```python
from build123d import *

# Parameters (mm, degrees)
SKETCH_1_W          = 100
SKETCH_1_H          = 53
SKETCH_1_W_2        = 30
SKETCH_1_H_2        = 43
SKETCH_1_W_3        = 50
SKETCH_1_H_3        = 25
SKETCH_1_H_4        = 10
EXTRUDE_1_DEPTH     = 7
FILLET_1_R          = 1
CUT_EXTRUDE_2_REACH = 115.393
SKETCH_2_R          = 1.5
SKETCH_3_R          = 1
CUT_EXTRUDE_3_DEPTH = 5


with BuildPart() as part:
    # 草图1 → 凸台-拉伸1 (new body)
    with BuildSketch(Plane.XY):
        with Locations((50, 26.5)):
            Rectangle(SKETCH_1_W, SKETCH_1_H)
        with Locations((20, 26.5)):
            Rectangle(SKETCH_1_W_2, SKETCH_1_H_2, mode=Mode.SUBTRACT)
        with Locations((70, 35.5)):
            Rectangle(SKETCH_1_W_3, SKETCH_1_H_3, mode=Mode.SUBTRACT)
        with Locations((70, 13)):
            Rectangle(SKETCH_1_W_3, SKETCH_1_H_4, mode=Mode.SUBTRACT)
    extrude(amount=EXTRUDE_1_DEPTH)

    # 圆角1
    fillet_1_edges = [part.edges().sort_by_distance(p)[0] for p in [
        (35, 48, 3.5),
        (5, 48, 3.5),
        (5, 5, 3.5),
        (35, 5, 3.5),
        (95, 48, 3.5),
        (45, 48, 3.5),
        (45, 23, 3.5),
        (95, 23, 3.5),
    ]]
    fillet(fillet_1_edges, radius=FILLET_1_R)

    # 草图2 → 切除-拉伸2 (cut, up to next)
    with BuildSketch(Plane.XZ, mode=Mode.PRIVATE) as cut_extrude_2_sk1:
        with Locations(Location((15, 3.5, 0), (0, 0, 270))):
            Circle(SKETCH_2_R)
    cut_extrude_2_tool1 = extrude(cut_extrude_2_sk1.sketch, amount=-CUT_EXTRUDE_2_REACH, mode=Mode.PRIVATE) & part.part
    # 草图2 → 切除-拉伸2 (cut, up to next)
    with BuildSketch(Plane.XZ, mode=Mode.PRIVATE) as cut_extrude_2_sk2:
        with Locations(Location((85, 3.5, 0), (0, 0, 270))):
            Circle(SKETCH_2_R)
    cut_extrude_2_tool2 = extrude(cut_extrude_2_sk2.sketch, amount=-CUT_EXTRUDE_2_REACH, mode=Mode.PRIVATE) & part.part
    # 草图2 → 切除-拉伸2 (cut, up to next)
    with BuildSketch(Plane.XZ, mode=Mode.PRIVATE) as cut_extrude_2_sk3:
        with Locations(Location((55, 3.5, 0), (0, 0, 270))):
            Circle(SKETCH_2_R)
    cut_extrude_2_tool3 = extrude(cut_extrude_2_sk3.sketch, amount=-CUT_EXTRUDE_2_REACH, mode=Mode.PRIVATE) & part.part
    # 草图2 → 切除-拉伸2 (cut, up to next)
    with BuildSketch(Plane.XZ, mode=Mode.PRIVATE) as cut_extrude_2_sk4:
        with Locations(Location((30, 3.5, 0), (0, 0, 270))):
            Circle(SKETCH_2_R)
    cut_extrude_2_tool4 = extrude(cut_extrude_2_sk4.sketch, amount=-CUT_EXTRUDE_2_REACH, mode=Mode.PRIVATE) & part.part
    add(cut_extrude_2_tool1.solids().sort_by_distance((15, 0, 3.5))[0], mode=Mode.SUBTRACT)
    add(cut_extrude_2_tool2.solids().sort_by_distance((85, 0, 3.5))[0], mode=Mode.SUBTRACT)
    add(cut_extrude_2_tool3.solids().sort_by_distance((55, 0, 3.5))[0], mode=Mode.SUBTRACT)
    add(cut_extrude_2_tool4.solids().sort_by_distance((30, 0, 3.5))[0], mode=Mode.SUBTRACT)

    # 草图3 → 切除-拉伸3 (cut)
    with BuildSketch(Plane(origin=(0, 53, 0), x_dir=(1, 0, 0), z_dir=(0, 1, 0))):
        with Locations(Location((80, -3.5, 0), (0, 0, 180))):
            Circle(SKETCH_3_R)
        with Locations(Location((65, -3.5, 0), (0, 0, 180))):
            Circle(SKETCH_3_R)
        with Locations(Location((20, -3.5, 0), (0, 0, 180))):
            Circle(SKETCH_3_R)
    extrude(amount=-CUT_EXTRUDE_3_DEPTH, mode=Mode.SUBTRACT)


solid = part.part
```
Geometry: final body of the model. Coordinates: model frame, mm. A direction names the side the tool comes from. Give positions to 0.01 mm unless a question says otherwise; leave off trailing zeros. Loops run counter-clockwise (first coordinate to the right, second up) from the corner with the lowest first, then second, coordinate; pieces in that order, holes last. Notation, with made-up numbers: (-34.5, 19) -> (-24.5, 19) arc R31 cw to (-24.5, 45) -> close; hole circle Ø10 at (78.25, 5.5). An arc over 180 degrees is marked (long way). Return JSON: item names as keys, results as strings.
Item 1: Pin query (flat end, axial travel): P1, Ø2, axis at y = 40.5, z = 3, coming from the -X side; P2, Ø1.6, axis at x = 65, z = 3.5, coming from the +Y side. Return the tip coordinate at first contact, or that it passes through.
Filled in:
{"P1": "x = 0", "P2": "y = 23"}
Item 2: Line query: line 1 (Y direction, x = 57.5, z = 3); line 2 (X direction, y = 11, z = 1); line 3 (X direction, y = 2.75, z = 3.5). Output: solid intervals per line, ascending.
Filled in:
{"line 1": "0 to 8, 18 to 23, 48 to 53", "line 2": "0 to 5, 35 to 45, 95 to 100", "line 3": "0 to 13.5, 16.5 to 28.5, 31.5 to 53.5, 56.5 to 83.5, 86.5 to 100"}
Item 3: Section B-B, the plane y = 46. Output: boundary loops of the cut face in (x, z), plus the area to 3 significant figures.
Filled in:
{"outline": "(0, 0) -> (5, 0) -> (5, 7) -> (0, 7) -> close; (35, 0) -> (45, 0) -> (45, 7) -> (35, 7) -> close; (95, 0) -> (100, 0) -> (100, 7) -> (95, 7) -> close", "area": "140 mm^2"}
Item 4: Mould query, pull axis X, two halves, no side actions, for faces 1 (the flat face through (100, 26, 3)), 2 (the flat face through (0, 26, 3)), 3 (the flat face through (95, 13, 3)), 4 (the flat face through (38, 27, 7)). Classes: released by +X, released by -X, zero draft, split by the parting line, or undercut.
Filled in:
{"face 1": "released by +X", "face 2": "released by -X", "face 3": "undercut", "face 4": "zero draft"}
Item 5: Access query for faces 5 (the cylindrical face through (15, 2, 2)), 6 (the flat face through (20, 5, 3)), 7 (the cylindrical face through (21, 50.5, 3.5)). Directions: +Z, -Z, +X, -X, +Y, -Y. A direction counts if a zero-diameter tool reaches every point of the face in a straight line with its end or side. Return the directions, or none.
Filled in:
{"face 5": "-Y", "face 6": "+Z, -Z", "face 7": "+Y"}
Item 6: Section A-A, the plane x = 80. Output: boundary loops of the cut face in (y, z).
Filled in:
{"outline": "(0, 0) -> (8, 0) -> (8, 7) -> (0, 7) -> close; (18, 0) -> (23, 0) -> (23, 7) -> (18, 7) -> close; (48, 0) -> (53, 0) -> (53, 2.5) -> (48, 2.5) -> close; (48, 4.5) -> (53, 4.5) -> (53, 7) -> (48, 7) -> close"}
Item 7: Section C-C, the plane x = 59. Output: boundary loops of the cut face in (y, z), plus the area to 3 significant figures.
Filled in:
{"outline": "(0, 0) -> (8, 0) -> (8, 7) -> (0, 7) -> close; (18, 0) -> (23, 0) -> (23, 7) -> (18, 7) -> close; (48, 0) -> (53, 0) -> (53, 7) -> (48, 7) -> close", "area": "126 mm^2"}
